Could you check a few things on this model? Use its own coordinates, in mm. Give positions to 0.01 mm unless a question says otherwise; leave off trailing zeros. Loops run counter-clockwise (first coordinate to the right, second up) from the corner with the lowest first, then second, coordinate; pieces in that order, holes last. Notation, with made-up numbers: (-16.5, 65.5) -> (41.5, 65.5) arc R16 ccw to (41.5, 82.5) -> close; hole circle Ø11 at (25, 51.5). An arc over 180 degrees is marked (long way). Put each result on its own line as item: value.
```python
from build123d import *

# Parameters (mm, degrees)
F0_W     = 431.8
F0_H     = 254
F0_R     = 12.7
F1_DEPTH = 22.225


with BuildPart() as f1:
    # F0 (on Top) → F1 (new body)
    with BuildSketch(Plane.XY):
        Rectangle(F0_W, F0_H)
        with Locations((-174.625, -85.725)):
            Circle(F0_R, mode=Mode.SUBTRACT)
        with Locations((0, -85.725)):
            Circle(F0_R, mode=Mode.SUBTRACT)
        with Locations((174.625, -85.725)):
            Circle(F0_R, mode=Mode.SUBTRACT)
        with Locations((-174.625, 85.725)):
            Circle(F0_R, mode=Mode.SUBTRACT)
        with Locations((0, 85.725)):
            Circle(F0_R, mode=Mode.SUBTRACT)
        with Locations((174.625, 85.725)):
            Circle(F0_R, mode=Mode.SUBTRACT)
    extrude(amount=F1_DEPTH)


solid = f1.part
```
1. If we section it at C-C (z = 12.5): List the corners of the cut face in (x, y) for me (3 decimals).
Recorded:
outline: (-215.9, -127) -> (215.9, -127) -> (215.9, 127) -> (-215.9, 127) -> close; hole circle Ø25.4 at (-174.625, -85.725); hole circle Ø25.4 at (-174.625, 85.725); hole circle Ø25.4 at (0, -85.725); hole circle Ø25.4 at (0, 85.725); hole circle Ø25.4 at (174.625, -85.725); hole circle Ø25.4 at (174.625, 85.725)
2. I need wall thicknesses on line 1 (Y direction, x = 0, z = 17.5) (3 decimals); line 2 (X direction, y = -78.5, z = 2.75); line 3 (X direction, y = -78, z = 19.5). Which ranges of each line are inside material? Lowest first, please.
Recorded:
line 1: y = -127 to -98.425, -73.025 to 73.025, 98.425 to 127
line 2: x = -215.9 to -185.07, -164.18 to -10.44, 10.44 to 164.18, 185.07 to 215.9
line 3: x = -215.9 to -184.71, -164.54 to -10.08, 10.08 to 164.54, 184.71 to 215.9
3. If we section it at B-B (y = 90): List the corners of the cut face in (x, z) for me (3 decimals).
Recorded:
outline: (-215.9, 0) -> (-186.584, 0) -> (-186.584, 22.225) -> (-215.9, 22.225) -> close; (-162.666, 0) -> (-11.959, 0) -> (-11.959, 22.225) -> (-162.666, 22.225) -> close; (11.959, 0) -> (162.666, 0) -> (162.666, 22.225) -> (11.959, 22.225) -> close; (186.584, 0) -> (215.9, 0) -> (215.9, 22.225) -> (186.584, 22.225) -> close
4. Thinking about a two-plate mould opening in X: for faces 1 (the face through (-162.5, 89.5, 11)), 2 (the face through (-3, 2, 0)), 3 (the face through (-1.653, -73.133, 10.957)), 4 (the face through (-215.9, -2, 11)), which applies, pulls with the +X half, pulls with the -X half, needs draft (parallel to the pull), parting line crosses it, or undercut?
Recorded:
face 1: undercut
face 2: needs draft
face 3: undercut
face 4: pulls with the -X half
5. If we section it at A-A (x = 0): List the corners of the cut face in (y, z) for me (3 decimals).
Recorded:
outline: (-127, 0) -> (-98.425, 0) -> (-98.425, 22.225) -> (-127, 22.225) -> close; (-73.025, 0) -> (73.025, 0) -> (73.025, 22.225) -> (-73.025, 22.225) -> close; (98.425, 0) -> (127, 0) -> (127, 22.225) -> (98.425, 22.225) -> close
6. I'm going to push flat-ended pins straight in: pin 1 (15 mm diameter, centred on x = 174.625, y = -85.725, fed in from -Z); pin 2 (8 mm diameter, centred on x = -134, y = 5, fed in from -Z). Where does each tip first touch, or does it pass through?
Recorded:
pin 1: passes through
pin 2: stops at z = 0
